```python
from build123d import *

# Parameters (mm, degrees)
BOSS_EXTRUDE1_DEPTH         = 2.54
SKETCH6_R                   = 2.9845
SKETCH6_W                   = 20.32
SKETCH6_H                   = 25.4
SKETCH6_H_2                 = 8.636
CUT_EXTRUDE1_DEPTH          = 3.54
F_27_0_144_DIAMETER_HOLE1_D = 3.6576


with BuildPart() as part:
    # Sketch1 → Boss-Extrude1 (new body)
    with BuildSketch(Plane(origin=(0, 0, 0), x_dir=(0, 1, 0), z_dir=(0, 0, 1))):
        with BuildLine():
            Line((-97.2566, -88.9), (97.2566, -88.9))
            ThreePointArc((97.2566, -88.9), (109.308103714, -83.908103714), (114.3, -71.8566))
            Line((114.3, -71.8566), (114.3, 71.8566))
            ThreePointArc((114.3, 71.8566), (109.308103714, 83.908103714), (97.2566, 88.9))
            Line((97.2566, 88.9), (-97.2566, 88.9))
            ThreePointArc((-97.2566, 88.9), (-109.308103714, 83.908103714), (-114.3, 71.8566))
            Line((-114.3, 71.8566), (-114.3, -71.8566))
            ThreePointArc((-114.3, -71.8566), (-109.308103714, -83.908103714), (-97.2566, -88.9))
        make_face()
    extrude(amount=BOSS_EXTRUDE1_DEPTH)

    # Sketch6 → Cut-Extrude1 (cut, through all)
    with BuildSketch(Plane.XY.offset(2.54)):
        with Locations((58.279140867, 84.504640867)):
            Circle(SKETCH6_R)
        with Locations((58.279140867, 74.626359133)):
            Circle(SKETCH6_R)
        with Locations((48.400859133, 74.626359133)):
            Circle(SKETCH6_R)
        with Locations((48.400859133, 84.504640867)):
            Circle(SKETCH6_R)
        with Locations((-38.1, 76.835)):
            Circle(SKETCH6_R)
        with Locations((-31.115, 69.85)):
            Circle(SKETCH6_R)
        with Locations((-38.1, 62.865)):
            Circle(SKETCH6_R)
        with Locations((-45.085, 69.85)):
            Circle(SKETCH6_R)
        with Locations((53.34, 55.4355)):
            Rectangle(SKETCH6_W, SKETCH6_H)
        with Locations((53.34, 95.3135)):
            Rectangle(SKETCH6_W, SKETCH6_H_2)
    extrude(amount=-CUT_EXTRUDE1_DEPTH, mode=Mode.SUBTRACT)

    # #27 (0.144) Diameter Hole1 (through all)
    with Locations(Plane.XY.offset(2.54)):
        with Locations((69.21913, 99.508615), (69.21913, -99.508615), (-69.21913, 99.508615), (-69.21913, -99.508615)):
            Hole(F_27_0_144_DIAMETER_HOLE1_D / 2)


solid = part.part
```
Can you work these out from the model? Positions are in its coordinate system, mm. Give positions to 0.01 mm unless a question says otherwise; leave off trailing zeros. Loops run counter-clockwise (first coordinate to the right, second up) from the corner with the lowest first, then second, coordinate; pieces in that order, holes last. Notation, with made-up numbers: M 77,-28.5 L 94,-28.5 A17 cw 94,-15.5 Z; hole C 44,34 d7. An arc over 180 degrees is marked long. One line per question, with ' | ' between items. Start each with the question number.
Q1. If we section it at A-A (x = -38.1): Please give me the cut outline in (y, z).
Q2. If we section it at B-B (z = 0.5): State how many separate pieces and enclosed holes the cut face has, plus the area to 3 significant figures.
Q3. If we mould it in two halves opening along Y, with no side actions, what happens to faces 1 (the cylindrical face through (83.775, -109.44, 1.252)), 2 (the cylindrical face through (45.42, 84.64, 1.29)), 3 (the flat face through (-1, -2, 0)), 4 (the cylindrical face through (-83.775, 109.44, 1.252))? For each: +Y half, -Y half, draft (parallel to the pull), parting line (faces both ways), or undercut.
Q4. For pin 1 Ø5 at (x, y) = (58.28, 74.63) entering from +Z, with a flat end and sliding along its axis, tell me the tip position at first contact or that it passes through.
Q5. If I drill on line 1 (Y direction, x = -38.1, z = 0.9); line 2 (Y direction, x = 61, z = 2.05); line 3 (X direction, y = 48, z = 0.55), over which ranges is the centre line in solid material (lowest first)? Write a range as from..to.
Computed:
1) outline: M -114.3,0 L 59.88,0 L 59.88,2.54 L -114.3,2.54 Z; M 65.85,0 L 73.85,0 L 73.85,2.54 L 65.85,2.54 Z; M 79.82,0 L 114.3,0 L 114.3,2.54 L 79.82,2.54 Z
2) separate pieces: 1 | enclosed holes: 14 | area: 39,400 mm²
3) face 1: -Y half | face 2: undercut | face 3: draft | face 4: +Y half
4) pin 1: passes through
5) line 1: y = -114.3..59.88, 65.85..73.85, 79.82..114.3 | line 2: y = -114.3..42.74, 68.14..73.4, 75.85..83.28, 85.73..91, 99.63..114.3 | line 3: x = -88.9..43.18, 63.5..88.9
